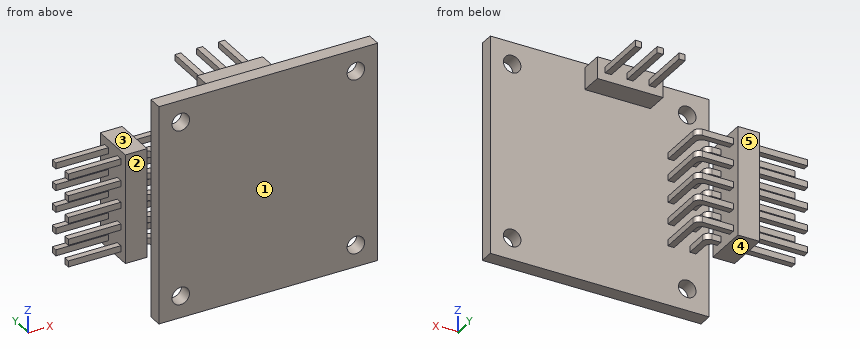
```python
from build123d import *

# Parameters (mm, degrees)
SKETCH1_W                = 25
SKETCH1_H                = 25
SKETCH1_R                = 1
BOSS_EXTRUDE1_DEPTH      = 1.6
BOSS_EXTRUDE2_START      = -7.5
BOSS_EXTRUDE2_DEPTH      = 0.7
LPATTERN1_COUNT          = 5
LPATTERN1_PITCH          = 2.5
BOSS_EXTRUDE3_DEPTH      = 0.9
BOSS_EXTRUDE3_DEPTH_BACK = 11.6
SKETCH4_W                = 2.5
SKETCH4_H                = 5
SKETCH5_W                = 2.5
SKETCH5_H                = 2.5
BOSS_EXTRUDE4_DEPTH      = 2.5
SKETCH6_W                = 0.7
SKETCH6_H                = 0.7
BOSS_EXTRUDE5_DEPTH      = 6
LPATTERN2_COUNT          = 3
LPATTERN2_PITCH          = 2.5


with BuildPart() as part:
    # Sketch1 → Boss-Extrude1 (new body)
    with BuildSketch(Plane(origin=(0, 0, 0), x_dir=(1, 0, 0), z_dir=(0, 1, 0))):
        with Locations((12.5, 12.5)):
            Rectangle(SKETCH1_W, SKETCH1_H)
        with Locations(Location((2.5, 22.5, 0), (0, 0, 270))):
            Circle(SKETCH1_R, mode=Mode.SUBTRACT)
        with Locations(Location((22.5, 22.5, 0), (0, 0, 270))):
            Circle(SKETCH1_R, mode=Mode.SUBTRACT)
        with Locations(Location((22.5, 2.5, 0), (0, 0, 270))):
            Circle(SKETCH1_R, mode=Mode.SUBTRACT)
        with Locations(Location((2.5, 2.5, 0), (0, 0, 270))):
            Circle(SKETCH1_R, mode=Mode.SUBTRACT)
    extrude(amount=BOSS_EXTRUDE1_DEPTH)

    # Sketch3 → Boss-Extrude2 (add)
    with BuildSketch(Plane.XY.offset(BOSS_EXTRUDE2_START)):
        with BuildLine():
            Line((1.5, 1.6), (1.5, 3.4))
            ThreePointArc((1.5, 3.4), (1.294974747, 3.894974747), (0.8, 4.1))
            Line((0.8, 4.1), (-8, 4.1))
            Line((-8, 4.1), (-8, 4.8))
            Line((-8, 4.8), (1.5, 4.8))
            ThreePointArc((1.5, 4.8), (1.994974747, 4.594974747), (2.2, 4.1))
            Line((2.2, 4.1), (2.2, 1.6))
            Line((2.2, 1.6), (1.5, 1.6))
        make_face()
        with BuildLine():
            Line((4, 1.6), (4.7, 1.6))
            Line((4.7, 1.6), (4.7, 6.6))
            ThreePointArc((4.7, 6.6), (4.494974747, 7.094974747), (4, 7.3))
            Line((4, 7.3), (-8, 7.3))
            Line((-8, 7.3), (-8, 6.6))
            Line((-8, 6.6), (3.3, 6.6))
            ThreePointArc((3.3, 6.6), (3.794974747, 6.394974747), (4, 5.9))
            Line((4, 5.9), (4, 1.6))
        make_face()
    boss_extrude2 = extrude(amount=-BOSS_EXTRUDE2_DEPTH)

    # LPattern1: Boss-Extrude2 ×5
    with Locations(*[(0, 0, -i * LPATTERN1_PITCH) for i in range(1, LPATTERN1_COUNT)]):
        add(boss_extrude2)

    # Sketch4 → Boss-Extrude3 (add, two sides: drawn at the far end of the back side and taken through both)
    with BuildSketch(Plane.XY.offset(-7.5).offset(-BOSS_EXTRUDE3_DEPTH_BACK)):
        with Locations((-0.75, 5.7)):
            Rectangle(SKETCH4_W, SKETCH4_H)
    extrude(amount=BOSS_EXTRUDE3_DEPTH + BOSS_EXTRUDE3_DEPTH_BACK)

    # Sketch5 → Boss-Extrude4 (add)
    with BuildSketch(Plane(origin=(0, 1.6, 0), x_dir=(1, 0, 0), z_dir=(0, 1, 0))):
        with Locations((7.95, 1.75)):
            Rectangle(SKETCH5_W, SKETCH5_H)
    boss_extrude4 = extrude(amount=BOSS_EXTRUDE4_DEPTH)

    # Sketch6 → Boss-Extrude5 (add)
    with BuildSketch(Plane(origin=(0, 4.1, 0), x_dir=(1, 0, 0), z_dir=(0, 1, 0))):
        with Locations((7.95, 1.75)):
            Rectangle(SKETCH6_W, SKETCH6_H)
    boss_extrude5 = extrude(amount=BOSS_EXTRUDE5_DEPTH)

    # LPattern2: Boss-Extrude4, Boss-Extrude5 ×3
    with Locations(*[(i * LPATTERN2_PITCH, 0, 0) for i in range(1, LPATTERN2_COUNT)]):
        add(boss_extrude4)
        add(boss_extrude5)


solid = part.part
```
The model under review builds one solid part; all positions refer to its coordinate system, in mm. Face numbers are marked on the shaded views. A direction names the side the tool comes from. Round coordinates to 2 decimals unless told otherwise and drop trailing zeros. Loops run counter-clockwise (first coordinate to the right, second up) from the corner with the lowest first, then second, coordinate; pieces in that order, holes last. Notation, with made-up numbers: (8.5, -2.75) -> (40.5, -2.75) arc R10 cw to (40.5, 6.25) -> close; hole circle Ø7 at (6, 28). An arc over 180 degrees is marked (long way). Answer in a Markdown table with one row per item.
1) For pin 1 Ø1 at (x, z) = (-1, -7) entering from +Y; pin 2 Ø0.6 at (x, y) = (-4.5, 4.5) entering from +Z; pin 3 Ø1 at (x, z) = (11, -21.5) entering from +Y, all flat-tipped, find the tip position at first contact; note any pin that passes through.
Taken from the geometry:
| item | result |
|---|---|
| pin 1 | stops at y = 8.2 |
| pin 2 | stops at z = -7.5 |
| pin 3 | stops at y = 1.6 |
2) Tool access review of the marked faces 1, 2, 3, 4 and 5: name each direction out of +Z, -Z, +X, -X, +Y, -Y from which nothing blocks a thin tool from reaching the whole face with its end or side.
Taken from the geometry:
| item | result |
|---|---|
| face 1 | +Z, -Z, +X, -X, -Y |
| face 2 | +Z, -Z, -X |
| face 3 | +Z, +X, -X, +Y |
| face 4 | -Z, +X, -X, +Y |
| face 5 | +Z, -Z, +X, -X, +Y |
3) Consider section A-A, the plane z = -2.5. Write out the cut boundary in (x, y), plus the area to 4 significant figures.
Taken from the geometry:
| item | result |
|---|---|
| outline | (0, 0) -> (1.5, 0) -> (1.5, 1.6) -> (0, 1.6) -> close; (3.5, 0) -> (21.5, 0) -> (21.5, 1.6) -> (14.2, 1.6) -> (14.2, 4.1) -> (6.7, 4.1) -> (6.7, 1.6) -> (3.5, 1.6) -> close; (23.5, 0) -> (25, 0) -> (25, 1.6) -> (23.5, 1.6) -> close |
| area | 52.35 mm² |
4) Consider section D-D, the plane y = 5.5. Count the separate pieces of the cut face and the enclosed holes in it, plus the area to 3 significant figures.
Taken from the geometry:
| item | result |
|---|---|
| separate pieces | 9 |
| enclosed holes | 0 |
| area | 35.2 mm² |
5) Consider section B-B, the plane z = -13.75. Write out the cut boundary in (x, y).
Taken from the geometry:
| item | result |
|---|---|
| outline | (-2, 3.2) -> (0.5, 3.2) -> (0.5, 8.2) -> (-2, 8.2) -> close; (0, 0) -> (25, 0) -> (25, 1.6) -> (0, 1.6) -> close |
6) Consider section C-C, the plane y = 1. Write out the cut boundary in (x, z).
Taken from the geometry:
| item | result |
|---|---|
| outline | (0, -25) -> (25, -25) -> (25, 0) -> (0, 0) -> close; hole circle Ø2 at (2.5, -22.5); hole circle Ø2 at (2.5, -2.5); hole circle Ø2 at (22.5, -22.5); hole circle Ø2 at (22.5, -2.5) |
7) Wall thickness on line 1 along X through (y, z) = (0.75, -2.5); line 2 along Y through (x, z) = (21, -6); line 3 along Y through (x, z) = (-1.5, -14.75): over which ranges is each line inside the solid? List them lowest first.
Taken from the geometry:
| item | result |
|---|---|
| line 1 | x = 0 to 1.5, 3.5 to 21.5, 23.5 to 25 |
| line 2 | y = 0 to 1.6 |
| line 3 | y = 3.2 to 8.2 |
